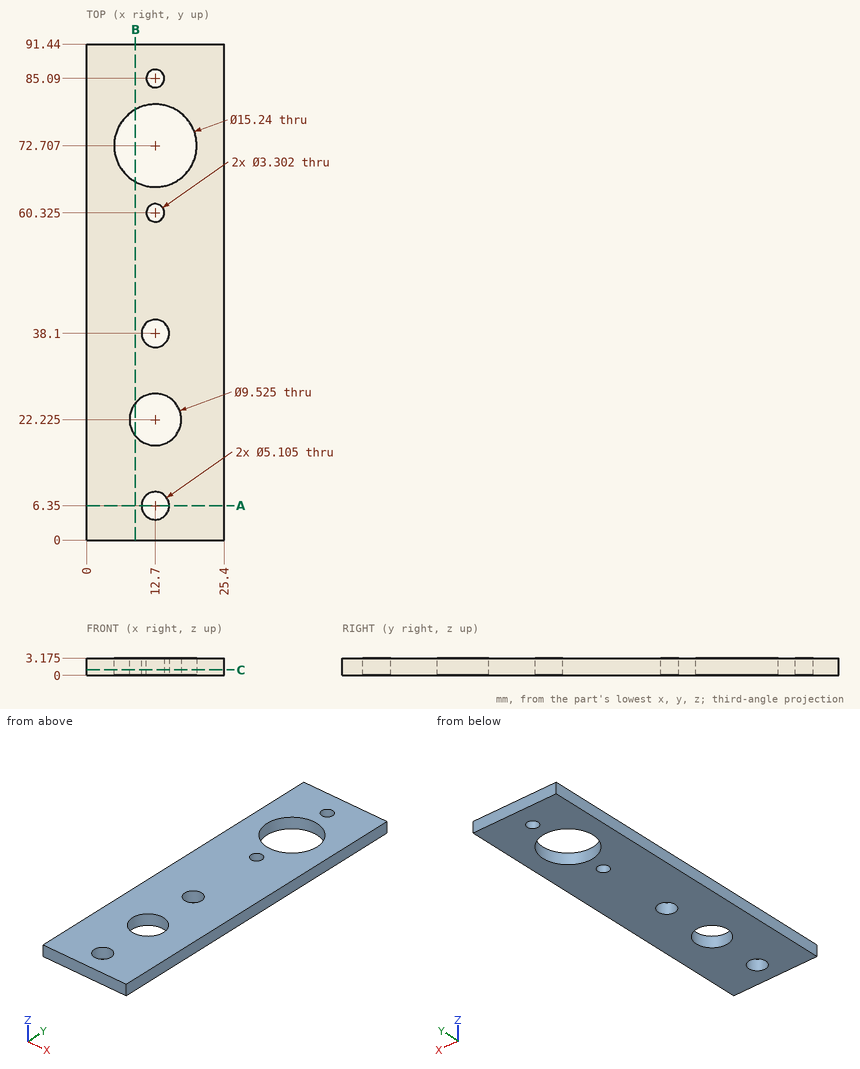
Here's the drawing with two shaded views (mm, measured from the low corner). I have some questions. Round coordinates to 2 decimals unless told otherwise and drop trailing zeros. Loops run counter-clockwise (first coordinate to the right, second up) from the corner with the lowest first, then second, coordinate; pieces in that order, holes last.
Item 1: Please list where these lines run through material, in increasing order: L1, parallel to X at y = 76, z = 1.4; L2, parallel to Y at x = 17.5, z = 2.4 (1 decimal); L3, parallel to X at y = 8.5, z = 1.25 (1 decimal).
Item 2: Suppose I cut it at A-A, the plane y = 6.35. Write out the boundary of the cut face in (x, z) (1 decimal).
Item 3: Suppose I cut it at B-B, the plane x = 9. Write out the boundary of the cut face in (y, z) (1 decimal), then the cut area to 3 significant figures.
Item 4: Suppose I cut it at C-C, the plane z = 1. State how many separate pieces and enclosed holes the cut face has, then the cut area to 3 significant figures.
Reported:
1. L1: x = 0 to 5.83, 19.57 to 25.4
1. L2: y = 0 to 66.8, 78.6 to 91.4
1. L3: x = 0 to 11.3, 14.1 to 25.4
2. outline: (0, 0) - (10.1, 0) - (10.1, 3.2) - (0, 3.2) - close; (15.3, 0) - (25.4, 0) - (25.4, 3.2) - (15.3, 3.2) - close
3. outline: (0, 0) - (19.2, 0) - (19.2, 3.2) - (0, 3.2) - close; (25.2, 0) - (66, 0) - (66, 3.2) - (25.2, 3.2) - close; (79.4, 0) - (91.4, 0) - (91.4, 3.2) - (79.4, 3.2) - close
3. area: 229 mm2
4. separate pieces: 1
4. enclosed holes: 6
4. area: 2,010 mm2
